Autodesk Inventor part; units mm, degrees
ref_plane "YZ Plane" through (0, 0, 0) normal (1, 0, 0) x (0, 1, 0)
ref_plane "XZ Plane" through (0, 0, 0) normal (0, 1, 0) x (-1, 0, 0)
ref_plane "XY Plane" through (0, 0, 0) normal (0, 0, 1) x (1, 0, 0)
sketch "Sketch1" plane through (0, 0, 0) normal (1, 0, 0) x (0, 1, 0)
  line L0 (0, 0) -> (6.5, 0)
  line L1 (6.5, 0) -> (6.5, -9)
  line L2 (6.5, -9) -> (0, -9)
  line L3 (0, -9) -> (0, 0)
  dimension "d0" = 6.5
  dimension "d1" = 9
extrude "Extrusion1" add sketch "Sketch1" along normal blind 350
sketch "Sketch2" plane through (350, 0, 0) normal (1, 0, 0) x (0, 0, -1)
  line L0 (0, 6.5) -> (0, 0)
  line L1 (0, 0) -> (9, 0) construction
  line L2 (9, 0) -> (9, 6.5)
  line L3 (9, 6.5) -> (0, 6.5) construction
  line L4 (0, 3) -> (1.25, 4.25)
  line L5 (1.25, 4.25) -> (0, 5.5)
  line L6 (9, 6.5) -> (0, 6.5)
  line L7 (4.5, 6.5) -> (4.5, 0) construction
  line L8 (0, 0) -> (9, 0)
  line L9 (9, 3) -> (7.75, 4.25)
  line L10 (7.75, 4.25) -> (9, 5.5)
  line L11 (9, 5.5) -> (9, 3)
  line L12 (9, 0) -> (9, 6.5)
  dimension "d4" = 3.5
  dimension "d5" = 1
  dimension "d6" = 45
extrude "Extrusion2" cut sketch "Sketch2" against normal through all contours L5 L4 L0 | L2 L9 L10
chamfer "Chamfer1" distance 0.5 angle 45 4 edges at (175, 6.5, 0) (175, 6.5, -9) (175, 4.25, -7.75) (175, 4.25, -1.25)
sketch "Sketch3" plane through (0, 6.5, -0.5) normal (0, 1, 0) x (1, 0, 0)
  line L0 (0, 8) -> (350, 8)
  line L1 (0, 0) -> (0, 8)
  line L2 (350, 0) -> (0, 0)
  line L3 (350, 8) -> (350, 0)
  line L4 (0, 4) -> (5, 4)
  circle A0 centre (5, 4) radius 1.75
  circle A1 centre (5, 4) radius 3
  point P0 (0, -0.5)
  dimension "d12" = 3.5
  dimension "d13" = 5
  dimension "d14" = 6
extrude "Extrusion3" cut sketch "Sketch3" against normal through all contours A0
extrude "Extrusion4" cut sketch "Sketch3" against normal blind 3.5 contours A1
pattern_linear "Rectangular Pattern1" count 18 spacing 20 along (1, 0, 0) of "Extrusion3", "Extrusion4"
properties part number "mgn9_350mm"
Source: CAD feature listing. Evaluate the final solid. Frame: model axes, mm. A direction names the side the tool comes from. Round coordinates to 2 decimals unless told otherwise and drop trailing zeros.
Q1. Section A-A, the plane y = 1.75. State how many separate pieces and enclosed holes the cut face has, plus the area to 3 significant figures.
Q2. Ray query, line 1 (Z direction, x = 345, y = 4.3); line 2 (Z direction, x = 125, y = 2.1); line 3 (Z direction, x = 295.5, y = 4). Return the intervals inside material, ascending.
Q3. First-contact query: P1, Ø1, axis at x = 143.5, z = -6, coming from the +Y side; P2, Ø3, axis at x = 245, z = -4.5, coming from the +Y side. Flat tips, straight axial feed; report the tip coordinate or a pass-through.
Q4. Access query for faces 1 (the face through (173, 0, -5)), 2 (the face through (202, 4.8, -4.6)). Directions: +Z, -Z, +X, -X, +Y, -Y. A direction counts if a zero-diameter tool reaches every point of the face in a straight line with its end or side. Return the directions, or none.
Solutions:
1. separate pieces: 1
1. enclosed holes: 18
1. area: 2,980 mm2
2. line 1: z = -8.1 to -7.5, -1.5 to -0.9
2. line 2: z = -9 to -6.25, -2.75 to 0
2. line 3: z = -8.1 to -0.9
3. P1: stops at y = 3
3. P2: passes through
4. face 1: +Z, -Z, +X, -X, -Y
4. face 2: +Y
